from build123d import *

# Parameters (mm, degrees)
F1_DEPTH = 4.2
F2_R     = 0.5
F3_DEPTH = 1.5
F4_R     = 2.5
F5_DEPTH = 1
F6_R     = 2.25
F7_DEPTH = 2.4
F8_R     = 1.25
F9_DEPTH = 25


with BuildPart() as f1:
    # F0 (on Top) → F1 (new body)
    with BuildSketch(Plane.XY):
        with BuildLine():
            ThreePointArc((2.1, -2.8), (3.130495, -1.565248), (3.5, 0))
            ThreePointArc((3.5, 0), (3.130495, 1.565248), (2.1, 2.8))
            ThreePointArc((2.1, 2.8), (0, 3.5), (-2.1, 2.8))
            ThreePointArc((-2.1, 2.8), (-3.5, 0), (-2.1, -2.8))
            ThreePointArc((-2.1, -2.8), (0, -3.5), (2.1, -2.8))
        make_face()
    extrude(amount=F1_DEPTH)

    # F2 (on face) → F3 (join)
    with BuildSketch(Plane.XY.offset(4.2)):
        with BuildLine():
            Line((-2.1, 2.8), (-14.347362, 1.793958))
            ThreePointArc((-14.347362, 1.793958), (-16, 0), (-14.347362, -1.793958))
            Line((-14.347362, -1.793958), (-2.1, -2.8))
            ThreePointArc((-2.1, -2.8), (-3.5, 0), (-2.1, 2.8))
        make_face()
        with Locations((-14.5, 0)):
            Circle(F2_R, mode=Mode.SUBTRACT)
        with Locations((-12.5, 0)):
            Circle(F2_R, mode=Mode.SUBTRACT)
        with Locations((-10.5, 0)):
            Circle(F2_R, mode=Mode.SUBTRACT)
        with Locations((-8.5, 0)):
            Circle(F2_R, mode=Mode.SUBTRACT)
        with Locations((-6.5, 0)):
            Circle(F2_R, mode=Mode.SUBTRACT)
        with Locations((-4.5, 0)):
            Circle(F2_R, mode=Mode.SUBTRACT)
        with BuildLine():
            Line((2.1, -2.8), (14.347362, -1.793958))
            ThreePointArc((14.347362, -1.793958), (16, 0), (14.347362, 1.793958))
            Line((14.347362, 1.793958), (2.1, 2.8))
            ThreePointArc((2.1, 2.8), (3.5, 0), (2.1, -2.8))
        make_face()
        with Locations((4.5, 0)):
            Circle(F2_R, mode=Mode.SUBTRACT)
        with Locations((6.5, 0)):
            Circle(F2_R, mode=Mode.SUBTRACT)
        with Locations((8.5, 0)):
            Circle(F2_R, mode=Mode.SUBTRACT)
        with Locations((10.5, 0)):
            Circle(F2_R, mode=Mode.SUBTRACT)
        with Locations((12.5, 0)):
            Circle(F2_R, mode=Mode.SUBTRACT)
        with Locations((14.5, 0)):
            Circle(F2_R, mode=Mode.SUBTRACT)
    extrude(amount=-F3_DEPTH)

    # F4 (on face) → F5 (cut)
    with BuildSketch(Plane.XY.offset(4.2)):
        Circle(F4_R)
    extrude(amount=-F5_DEPTH, mode=Mode.SUBTRACT)

    # F6 (on face) → F7 (cut)
    with BuildSketch(Plane(origin=(0, 0, 0), x_dir=(1, 0, 0), z_dir=(0, 0, -1))):
        Circle(F6_R)
    extrude(amount=-F7_DEPTH, mode=Mode.SUBTRACT)

    # F8 (on face) → F9 (cut)
    with BuildSketch(Plane.XY.offset(3.2)):
        Circle(F8_R)
    extrude(amount=-F9_DEPTH, mode=Mode.SUBTRACT)


solid = f1.part
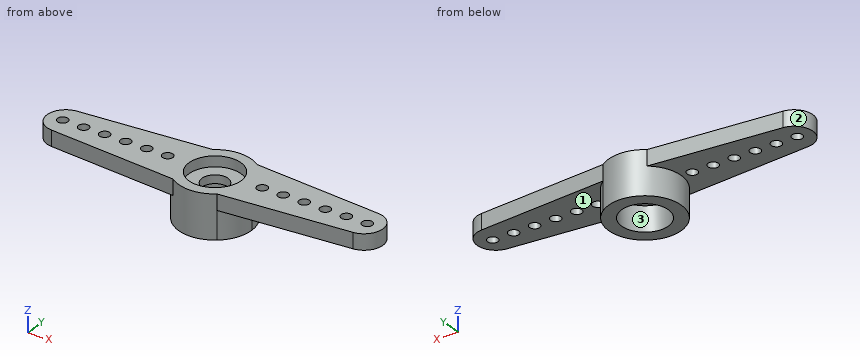
Input: part model. Units: mm. Frame: model coordinates. Face numbers are marked on the shaded views. Give positions to 0.01 mm unless a question says otherwise; leave off trailing zeros. Order: outer loops, then holes, each group sorted by start corner. A loop starts at its lowest first (then second) coordinate and runs counter-clockwise, first axis right, second up. Notation, with made-up numbers: (-20, 6) - (7, 6) arc R11 ccw to (7, 16) - close; hole circle Ø3 at (19, 35). An arc over 180 degrees is marked (long way). Answer as a JSON object with one key per item and string values. Group by question number.
Q1. Mould query, pull axis X, two halves, no side actions, for the marked faces 1, 2 and 3. Classes: pulls with the +X half, pulls with the -X half, needs draft (parallel to the pull), parting line crosses it, or undercut.
Q2. First-contact query: pin 1 Ø2 at (x, y) = (1, 1) entering from -Z; pin 2 Ø1.5 at (y, z) = (2, 1) entering from -X; pin 3 Ø3 at (x, y) = (9, 0) entering from -Z; pin 4 Ø3 at (x, y) = (0, 0) entering from +Z. Flat tips, straight axial feed; report the tip coordinate or a pass-through.
Q3. Cut plane C-C, the plane x = 6.5. Output: boundary loops of the cut face in (y, z).
Q4. Line query: probe 1 along Z at (x, y) = (-3.5, 1.25); probe 2 along Z at (x, y) = (-1.5, -0.5); probe 3 along Y at (x, z) = (-8.5, 3.95). Output: solid intervals per line, ascending.
Q5. Cut plane A-A, the plane x = -10.5. Output: boundary loops of the cut face in (y, z), then the cut area to 3 significant figures.
Q6. Cut plane B-B, the plane z = 1.85. Output: boundary loops of the cut face in (x, y).
Results:
{
 "1": {"face 1": "needs draft", "face 2": "pulls with the -X half", "face 3": "undercut"},
 "2": {"pin 1": "z = 0", "pin 2": "x = -3.27", "pin 3": "z = 2.7", "pin 4": "z = 3.2"},
 "3": {"outline": "(-2.44, 2.7) - (-0.5, 2.7) - (-0.5, 4.2) - (-2.44, 4.2) - close; (0.5, 2.7) - (2.44, 2.7) - (2.44, 4.2) - (0.5, 4.2) - close"},
 "4": {"probe 1": "2.7 to 4.2", "probe 2": "2.4 to 3.2", "probe 3": "-2.27 to -0.5, 0.5 to 2.27"},
 "5": {"outline": "(-2.11, 2.7) - (-0.5, 2.7) - (-0.5, 4.2) - (-2.11, 4.2) - close; (0.5, 2.7) - (2.11, 2.7) - (2.11, 4.2) - (0.5, 4.2) - close", "area": "4.83 mm^2"},
 "6": {"outline": "circle Ø7 at (0, 0); hole circle Ø4.5 at (0, 0)"}
}
